Source: CAD feature listing. Evaluate the final solid. Frame: model axes, mm. A direction names the side the tool comes from. Coordinates: 2 decimals unless noted, no trailing zeros. Loops run counter-clockwise (first coordinate to the right, second up) from the corner with the lowest first, then second, coordinate; pieces in that order, holes last. Notation, with made-up numbers: (67.5, 6.5) - (117.5, 6.5) arc R31 cw to (117.5, 40.5) - close; hole circle Ø2 at (60, 2.5). An arc over 180 degrees is marked (long way). Use CSV: the item, a comma, the result in double quotes. Start each with the question number.
Autodesk Inventor part; units mm, degrees
ref_plane "YZ Plane" through (0, 0, 0) normal (1, 0, 0) x (0, 1, 0)
ref_plane "XZ Plane" through (0, 0, 0) normal (0, 1, 0) x (-1, 0, 0)
ref_plane "XY Plane" through (0, 0, 0) normal (0, 0, 1) x (1, 0, 0)
sketch "Sketch1" plane through (0, 0, 0) normal (0, 0, 1) x (1, 0, 0)
  line L0 (-50, 10) -> (50, 10)
  line L1 (50, 10) -> (50, -10)
  line L2 (50, -10) -> (-50, -10)
  line L3 (-50, -10) -> (-50, 10)
  line L4 (-50, 10) -> (50, -10) construction
  line L5 (50, 10) -> (-50, -10) construction
  line L6 (51, 11) -> (-51, 11)
  line L7 (-51, 11) -> (-51, -11)
  line L8 (-51, -11) -> (51, -11)
  line L9 (51, -11) -> (51, 11)
  point P0 (0, 0)
  dimension "d0" = 100
  dimension "d1" = 20
  dimension "d2" = 1
extrude "Extrusion1" add sketch "Sketch1" along normal blind 2 contours L0 L1 L2 L3
extrude "Extrusion2" add sketch "Sketch1" along normal blind 4
properties part number "eit_chamber_solid_base"
(1) Pin query (flat end, axial travel): pin 1 Ø10 at (x, y) = (22.5, 1) entering from +Z. Return the tip coordinate at first contact, or that it passes through.
(2) Ray query, line 1 (Y direction, x = 17, z = 3.5); line 2 (X direction, y = -8, z = 2.3); line 3 (Z direction, x = -44, y = -8). Return the intervals inside material, ascending. Write a range as [from, to].
(3) Reachability of faces 1 (the flat face through (1, -10, 3)), 2 (the flat face through (51, 0, 2)) from +Z, -Z, +X, -X, +Y, -Y: full face, straight path, thin tool, end or side. Return the list, or none.
(4) Section C-C on y = 7. Output: boundary loops of the cut face in (x, z).
(5) Section B-B on x = -39. Output: boundary loops of the cut face in (y, z).
(6) Section A-A on z = 2.95. Output: boundary loops of the cut face in (x, y).
Solution:
1,pin 1,"stops at z = 2"
2,line 1,"y = [-11, -10], [10, 11]"
2,line 2,"x = [-51, -50], [50, 51]"
2,line 3,"z = [0, 2]"
3,face 1,"+Z"
3,face 2,"+Z, -Z, +X, +Y, -Y"
4,outline,"(-51, 0) - (51, 0) - (51, 4) - (50, 4) - (50, 2) - (-50, 2) - (-50, 4) - (-51, 4) - close"
5,outline,"(-11, 0) - (11, 0) - (11, 4) - (10, 4) - (10, 2) - (-10, 2) - (-10, 4) - (-11, 4) - close"
6,outline,"(-51, -11) - (51, -11) - (51, 11) - (-51, 11) - close; hole (-50, -10) - (50, -10) - (50, 10) - (-50, 10) - close"
